from build123d import *

# Parameters (mm, degrees)
EXTRUDE_1_DEPTH              = 3
HOLE_WIZARD_M5_1_D           = 4.2
HOLE_WIZARD_M5_1_CSINK_D     = 5.05
HOLE_WIZARD_M5_1_CSINK_ANGLE = 90
CUT_EXTRUDE_1_REACH          = 182.424
SKETCH_4_R                   = 4.1
FILLET_1_R                   = 10
CUT_EXTRUDE_2_REACH          = 182.424
SKETCH_5_R                   = 18
CUT_EXTRUDE_3_REACH          = 182.424


with BuildPart() as part:
    # 草图1 → 凸台-拉伸1 (new body)
    with BuildSketch(Plane(origin=(0, 0, 0), x_dir=(1, 0, 0), z_dir=(0, 1, 0))):
        with BuildLine():
            Line((0, 0), (70, 0))
            Line((70, 0), (70, -32.596529214))
            Line((70, -32.596529214), (83.512088558, -64.228012072))
            Line((83.512088558, -64.228012072), (108.512088558, -122.752426568))
            ThreePointArc((108.512088558, -122.752426568), (100.771987928, -142.036503054), (81.487911442, -134.296402424))
            Line((81.487911442, -134.296402424), (56.487911442, -75.771987928))
            Line((56.487911442, -75.771987928), (54.022278946, -70))
            Line((54.022278946, -70), (15.977721054, -70))
            Line((15.977721054, -70), (13.512088558, -75.771987928))
            Line((13.512088558, -75.771987928), (-11.487911442, -134.296402424))
            ThreePointArc((-11.487911442, -134.296402424), (-30.771987928, -142.036503054), (-38.512088558, -122.752426568))
            Line((-38.512088558, -122.752426568), (-13.512088558, -64.228012072))
            Line((-13.512088558, -64.228012072), (0, -32.596529214))
            Line((0, -32.596529214), (0, 0))
        make_face()
    extrude(amount=EXTRUDE_1_DEPTH)

    # M5 螺纹孔1 (through all)
    with Locations(Plane(origin=(0, 3, 0), x_dir=(1, 0, 0), z_dir=(0, 1, 0))):
        with Locations((9, -61), (61, -9), (9, -9), (61, -61)):
            CounterSinkHole(HOLE_WIZARD_M5_1_D / 2, HOLE_WIZARD_M5_1_CSINK_D / 2, counter_sink_angle=HOLE_WIZARD_M5_1_CSINK_ANGLE)

    # 草图4 → 切除-拉伸1 (cut, up to next)
    with BuildSketch(Plane(origin=(0, 3, 0), x_dir=(1, 0, 0), z_dir=(0, 1, 0)), mode=Mode.PRIVATE) as cut_extrude_1_sk1:
        with Locations(Location((-25, -128.524414496, 0), (0, 0, 270))):
            Circle(SKETCH_4_R)
    cut_extrude_1_tool1 = extrude(cut_extrude_1_sk1.sketch, amount=-CUT_EXTRUDE_1_REACH, mode=Mode.PRIVATE) & part.part
    # 草图4 → 切除-拉伸1 (cut, up to next)
    with BuildSketch(Plane(origin=(0, 3, 0), x_dir=(1, 0, 0), z_dir=(0, 1, 0)), mode=Mode.PRIVATE) as cut_extrude_1_sk2:
        with Locations(Location((95, -128.524414496, 0), (0, 0, 270))):
            Circle(SKETCH_4_R)
    cut_extrude_1_tool2 = extrude(cut_extrude_1_sk2.sketch, amount=-CUT_EXTRUDE_1_REACH, mode=Mode.PRIVATE) & part.part
    add(cut_extrude_1_tool1.solids().sort_by_distance((-25, 3, 128.524414))[0], mode=Mode.SUBTRACT)
    add(cut_extrude_1_tool2.solids().sort_by_distance((95, 3, 128.524414))[0], mode=Mode.SUBTRACT)

    # 圆角1
    fillet_1_edges = [part.edges().sort_by_distance(p)[0] for p in [
        (0, 1.5, 0),
        (70, 1.5, 0),
        (70, 1.5, 32.596529214),
        (54.022278946, 1.5, 70),
        (15.977721054, 1.5, 70),
        (0, 1.5, 32.596529214),
    ]]
    fillet(fillet_1_edges, radius=FILLET_1_R)

    # 草图5 → 切除-拉伸2 (cut, up to next)
    with BuildSketch(Plane(origin=(0, 3, 0), x_dir=(1, 0, 0), z_dir=(0, 1, 0)), mode=Mode.PRIVATE) as cut_extrude_2_sk1:
        with Locations(Location((35, -35, 0), (0, 0, 270))):
            Circle(SKETCH_5_R)
    cut_extrude_2_tool1 = extrude(cut_extrude_2_sk1.sketch, amount=-CUT_EXTRUDE_2_REACH, mode=Mode.PRIVATE) & part.part
    add(cut_extrude_2_tool1.solids().sort_by_distance((35, 3, 35))[0], mode=Mode.SUBTRACT)

    # 草图6 → 切除-拉伸3 (cut, up to next)
    with BuildSketch(Plane(origin=(0, 3, 0), x_dir=(1, 0, 0), z_dir=(0, 1, 0)), mode=Mode.PRIVATE) as cut_extrude_3_sk1:
        with BuildLine():
            Line((-22.485091694, -112.200038973), (-6.771815415, -75.415627212))
            ThreePointArc((-6.771815415, -75.415627212), (-1.390802391, -73.255835825), (0.768988996, -78.636848849))
            Line((0.768988996, -78.636848849), (-14.944287283, -115.42126061))
            ThreePointArc((-14.944287283, -115.42126061), (-20.325300307, -117.581051997), (-22.485091694, -112.200038973))
        make_face()
    cut_extrude_3_tool1 = extrude(cut_extrude_3_sk1.sketch, amount=-CUT_EXTRUDE_3_REACH, mode=Mode.PRIVATE) & part.part
    # 草图6 → 切除-拉伸3 (cut, up to next)
    with BuildSketch(Plane(origin=(0, 3, 0), x_dir=(1, 0, 0), z_dir=(0, 1, 0)), mode=Mode.PRIVATE) as cut_extrude_3_sk2:
        with BuildLine():
            Line((92.485091694, -112.200038973), (76.771815415, -75.415627212))
            ThreePointArc((76.771815415, -75.415627212), (71.390802391, -73.255835825), (69.231011004, -78.636848849))
            Line((69.231011004, -78.636848849), (84.944287283, -115.42126061))
            ThreePointArc((84.944287283, -115.42126061), (90.325300307, -117.581051997), (92.485091694, -112.200038973))
        make_face()
    cut_extrude_3_tool2 = extrude(cut_extrude_3_sk2.sketch, amount=-CUT_EXTRUDE_3_REACH, mode=Mode.PRIVATE) & part.part
    # 草图6 → 切除-拉伸3 (cut, up to next)
    with BuildSketch(Plane(origin=(0, 3, 0), x_dir=(1, 0, 0), z_dir=(0, 1, 0)), mode=Mode.PRIVATE) as cut_extrude_3_sk3:
        with BuildLine():
            Line((23, -6.522932736), (47, -6.522932736))
            ThreePointArc((47, -6.522932736), (49.477067264, -9), (47, -11.477067264))
            Line((47, -11.477067264), (23, -11.477067264))
            ThreePointArc((23, -11.477067264), (20.522932736, -9), (23, -6.522932736))
        make_face()
    cut_extrude_3_tool3 = extrude(cut_extrude_3_sk3.sketch, amount=-CUT_EXTRUDE_3_REACH, mode=Mode.PRIVATE) & part.part
    # 草图6 → 切除-拉伸3 (cut, up to next)
    with BuildSketch(Plane(origin=(0, 3, 0), x_dir=(1, 0, 0), z_dir=(0, 1, 0)), mode=Mode.PRIVATE) as cut_extrude_3_sk4:
        with BuildLine():
            Line((63.477067264, -23), (63.477067264, -47))
            ThreePointArc((63.477067264, -47), (61, -49.477067264), (58.522932736, -47))
            Line((58.522932736, -47), (58.522932736, -23))
            ThreePointArc((58.522932736, -23), (61, -20.522932736), (63.477067264, -23))
        make_face()
    cut_extrude_3_tool4 = extrude(cut_extrude_3_sk4.sketch, amount=-CUT_EXTRUDE_3_REACH, mode=Mode.PRIVATE) & part.part
    # 草图6 → 切除-拉伸3 (cut, up to next)
    with BuildSketch(Plane(origin=(0, 3, 0), x_dir=(1, 0, 0), z_dir=(0, 1, 0)), mode=Mode.PRIVATE) as cut_extrude_3_sk5:
        with BuildLine():
            Line((47, -63.477067264), (23, -63.477067264))
            ThreePointArc((23, -63.477067264), (20.522932736, -61), (23, -58.522932736))
            Line((23, -58.522932736), (47, -58.522932736))
            ThreePointArc((47, -58.522932736), (49.477067264, -61), (47, -63.477067264))
        make_face()
    cut_extrude_3_tool5 = extrude(cut_extrude_3_sk5.sketch, amount=-CUT_EXTRUDE_3_REACH, mode=Mode.PRIVATE) & part.part
    # 草图6 → 切除-拉伸3 (cut, up to next)
    with BuildSketch(Plane(origin=(0, 3, 0), x_dir=(1, 0, 0), z_dir=(0, 1, 0)), mode=Mode.PRIVATE) as cut_extrude_3_sk6:
        with BuildLine():
            Line((6.522932736, -47), (6.522932736, -23))
            ThreePointArc((6.522932736, -23), (9, -20.522932736), (11.477067264, -23))
            Line((11.477067264, -23), (11.477067264, -47))
            ThreePointArc((11.477067264, -47), (9, -49.477067264), (6.522932736, -47))
        make_face()
    cut_extrude_3_tool6 = extrude(cut_extrude_3_sk6.sketch, amount=-CUT_EXTRUDE_3_REACH, mode=Mode.PRIVATE) & part.part
    add(cut_extrude_3_tool1.solids().sort_by_distance((-10.858051, 3, 95.418444))[0], mode=Mode.SUBTRACT)
    add(cut_extrude_3_tool2.solids().sort_by_distance((80.858051, 3, 95.418444))[0], mode=Mode.SUBTRACT)
    add(cut_extrude_3_tool3.solids().sort_by_distance((35, 3, 9))[0], mode=Mode.SUBTRACT)
    add(cut_extrude_3_tool4.solids().sort_by_distance((61, 3, 35))[0], mode=Mode.SUBTRACT)
    add(cut_extrude_3_tool5.solids().sort_by_distance((35, 3, 61))[0], mode=Mode.SUBTRACT)
    add(cut_extrude_3_tool6.solids().sort_by_distance((9, 3, 35))[0], mode=Mode.SUBTRACT)


solid = part.part
CAD build for the part. Positions are in the model's coordinates, mm. A direction names the side the tool comes from. Coordinates: 2 decimals unless noted, no trailing zeros. Write each loop counter-clockwise with the first axis right and the second up, starting at its lowest first coordinate (ties: lowest second). Pieces come first, ordered by that corner, then holes. Notation, with made-up numbers: M 84,39 L 91,39 A14 ccw 91,45 Z; hole C -33.75,15 d1. An arc over 180 degrees is marked long. Answer as a JSON object with one key per item and string values. Group by question number.
1) Wall check: line 1 (X direction, y = 1.6, z = 84); line 2 (X direction, y = 0.2, z = 108.5); line 3 (Z direction, x = 61, y = 1.95). Give the ranges that are in metal, low to high. Write a range as from..to.
2) Tool access for faces 1 (the face through (66.99, 1.52, 2.85)), 2 (the face through (69.226, 1.479, 105.592)), 3 (the face through (-14.74, 1.52, 94.07)): list every direction of +Z, -Z, +X, -X, +Y, -Y with a clear straight run to the whole face (end or side of a thin tool).
3) Saw through at C-C (x = 95). Write the cut outline in (y, z), plus the area to 3 significant figures.
4) Saw through at B-B (z = 26). Write the cut outline in (x, y).
5) Mould opens along Z. For faces 4 (the face through (76.978, 1.521, 96.772)), 5 (the face through (84.74, 1.52, 94.07)), 6 (the face through (-30.47, 1.48, 142.16)), 7 (the face through (3.01, 1.52, 2.85)) say: +Z half, -Z half, draft (parallel to the pull), parting line (faces both ways), or undercut.
6) Pin check, flat tips, straight feed: pin 1 Ø1.5 at (y, z) = (2, 37.5) entering from +X (3 decimals); pin 2 Ø0.9 at (y, z) = (1, 34.5) entering from +X; pin 3 Ø1 at (x, y) = (23.5, 1.5) entering from +Z. Stop position of each tip, or through.
7) Saw through at D-D (y = 1.6). Give the number of separate pieces and of enclosed holes in the cut face, plus the area to 3 significant figures.
8) Saw through at A-A (x = 35). Write the cut outline in (y, z), plus the area to 3 significant figures.
Values follow:
{
 "1": {"line 1": "x = -21.96..-10.44, -1.52..10, 60..71.52, 80.44..91.96", "line 2": "x = -32.42..-20.9, -11.99..-0.47, 70.47..81.99, 90.9..102.42", "line 3": "z = 0.05..6.9, 11.1..20.52, 49.48..58.9, 63.1..86.33"},
 "2": {"face 1": "-Z, +X, +Y, -Y", "face 2": "+Z, +Y, -Y", "face 3": "+Y, -Y"},
 "3": {"outline": "M 0,91.12 L 3,91.12 L 3,124.42 L 0,124.42 Z; M 0,132.62 L 3,132.62 L 3,143.22 L 0,143.22 Z", "area": "132 mm2"},
 "4": {"outline": "M 0,0 L 6.52,0 L 6.52,3 L 0,3 Z; M 11.48,0 L 19.41,0 L 19.41,3 L 11.48,3 Z; M 50.59,0 L 58.52,0 L 58.52,3 L 50.59,3 Z; M 63.48,0 L 70,0 L 70,3 L 63.48,3 Z"},
 "5": {"face 4": "undercut", "face 5": "undercut", "face 6": "parting line", "face 7": "-Z half"},
 "6": {"pin 1": "stops at x = 72.415", "pin 2": "stops at x = 71.01", "pin 3": "stops at z = 70"},
 "7": {"separate pieces": "1", "enclosed holes": "13", "area": "7,400 mm2"},
 "8": {"outline": "M 0,0 L 3,0 L 3,6.52 L 0,6.52 Z; M 0,11.48 L 3,11.48 L 3,17 L 0,17 Z; M 0,53 L 3,53 L 3,58.52 L 0,58.52 Z; M 0,63.48 L 3,63.48 L 3,70 L 0,70 Z", "area": "72.3 mm2"}
}
